Autodesk Inventor part; units mm, degrees
ref_plane "YZ Plane" through (0, 0, 0) normal (1, 0, 0) x (0, 1, 0)
ref_plane "XZ Plane" through (0, 0, 0) normal (0, 1, 0) x (-1, 0, 0)
ref_plane "XY Plane" through (0, 0, 0) normal (0, 0, 1) x (1, 0, 0)
sketch "Sketch1" plane through (0, 0, 0) normal (0, 0, 1) x (1, 0, 0)
  circle A0 centre (0, 0) radius 14.2875
  dimension "d0" = 28.575
extrude "Extrusion1" add sketch "Sketch1" along normal blind 12.7
sketch "Sketch2" plane through (0, 0, 12.7) normal (0, 0, 1) x (1, 0, 0)
  circle A0 centre (0, 0) radius 14.2875
  circle A1 centre (0, 0) radius 6.35
  dimension "d4" = 12.7
extrude "Extrusion2" add sketch "Sketch2" along normal blind 6.35 contours A1
sketch "Sketch3" plane through (0, 0, 12.7) normal (0, 0, 1) x (1, 0, 0)
  circle A0 centre (0, 0) radius 6.35
  circle A1 centre (0, 0) radius 14.2875
  circle A2 centre (0, 0) radius 9.525
  dimension "d7" = 19.05
extrude "Extrusion3" cut sketch "Sketch3" against normal blind 0.127 contours A2
properties part number ".6250  Bearing Press"
Read the model definition and answer for the solid it produces. Units are mm, in the model's axes. A direction names the side the tool comes from. Coordinates: 2 decimals unless noted, no trailing zeros. Loops run counter-clockwise (first coordinate to the right, second up) from the corner with the lowest first, then second, coordinate; pieces in that order, holes last. Notation, with made-up numbers: (76.25, -34) -> (84.25, -34) arc R26 ccw to (84.25, -10) -> close; hole circle Ø5 at (45.5, 41). An arc over 180 degrees is marked (long way). Return JSON: item names as keys, results as strings.
Item 1: For a pull along Y with two mould halves and no side action, classify faces 1 (the cylindrical face through (-14.274, -0.628, 6.261)), 2 (the flat face through (3, -9.3, 12.7)), 3 (the flat face through (6.2, -2, 12.573)) as +Y half, -Y half, draft (parallel to the pull), parting line (faces both ways), or undercut.
Answers:
{"face 1": "parting line", "face 2": "draft", "face 3": "undercut"}
Item 2: For faces 4 (the cylindrical face through (-1.38, -6.2, 15.86)), 5 (the flat face through (0, 0, 0)), determine the directions among +Z, -Z, +X, -X, +Y, -Y from which every point of the face is accessible in a straight line to the end or side of a thin tool.
Answers:
{"face 4": "+Z", "face 5": "-Z, +X, -X, +Y, -Y"}
Item 3: Find section D-D (x = 9). Determine the outline of the cut face in (y, z), plus the area to 3 significant figures.
Answers:
{"outline": "(-11.1, 0) -> (11.1, 0) -> (11.1, 12.7) -> (3.12, 12.7) -> (3.12, 12.57) -> (-3.12, 12.57) -> (-3.12, 12.7) -> (-11.1, 12.7) -> close", "area": "281 mm2"}
Item 4: Find section C-C (z = 9). Determine the outline of the cut face in (x, y) (1 decimal).
Answers:
{"outline": "circle Ø28.6 at (0, 0)"}
Item 5: Flat-ended cylindrical pins translate along their axes: P1, Ø5, axis at x = -5, z = 11.5, coming from the -Y side; P2, Ø1.5, axis at x = 7.5, z = 10, coming from the +Y side; P3, Ø3, axis at y = 10, z = 9, coming from the +X side. Find the tip coordinate at first contact, or state that the pin passes through.
Answers:
{"P1": "stops at y = -14.07", "P2": "stops at y = 12.59", "P3": "stops at x = 11.48"}
Item 6: Find the intervals of material crossed by probe 1 along Z at (x, y) = (-1.25, 11.25); probe 2 along Z at (x, y) = (-2, 8); probe 3 along Y at (x, z) = (-3.75, 12), in increasing order.
Answers:
{"probe 1": "z = 0 to 12.7", "probe 2": "z = 0 to 12.57", "probe 3": "y = -13.79 to 13.79"}
